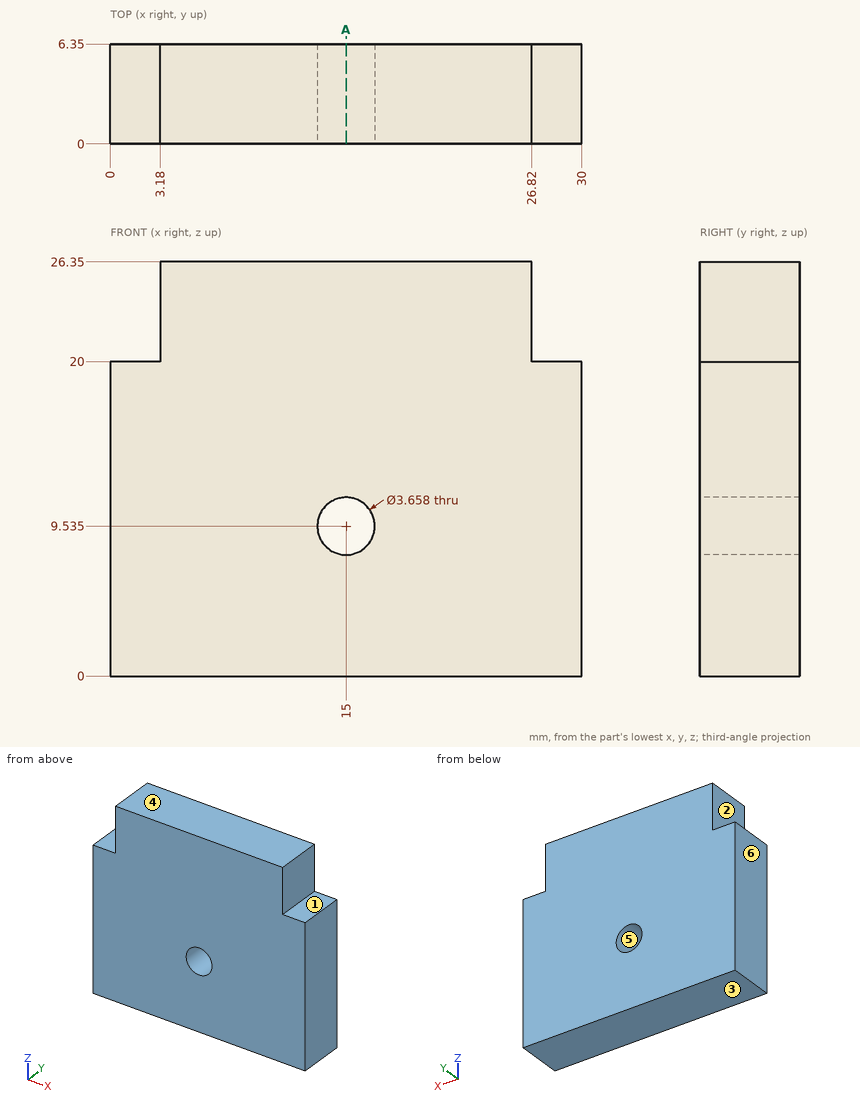
Drawing for the job (mm, zero at the part's lowest x, y, z). A direction names the side the tool comes from. Give positions to 0.01 mm unless a question says otherwise; leave off trailing zeros. Loops run counter-clockwise (first coordinate to the right, second up) from the corner with the lowest first, then second, coordinate; pieces in that order, holes last. Notation, with made-up numbers: (-28.5, 9.25) - (11.5, 9.25) arc R20 ccw to (11.5, 29.25) - close; hole circle Ø3 at (20.5, 33.5). An arc over 180 degrees is marked (long way). Write item = value, one per line. Start each with the question number.
1) Probe probe 1 along Z at (x, y) = (15, 1.5); probe 2 along X at (y, z) = (4.25, 24). List the from-to ranges inside material, lowest first. Write a range as from..to.
2) Pull direction Z, two halves, no side cores. Call the marked faces 4, 5 and 6: +Z half, -Z half, draft (parallel to the pull), parting line (faces both ways), or undercut.
3) Band-saw the part on A-A on x = 15. Give the cut face in (y, z).
4) Tool access for the marked faces 1, 2 and 3: list every direction of +Z, -Z, +X, -X, +Y, -Y with a clear straight run to the whole face (end or side of a thin tool).
5) Drop flat-ended pins along their axis: pin 1 Ø1 at (x, y) = (29, 3.5) entering from +Z; pin 2 Ø1.5 at (y, z) = (1.5, 21) entering from +X; pin 3 Ø1.9 at (y, z) = (3, 24.5) entering from -X. Give the stop position or say it passes through.
Final values:
q1.probe_1 = 0..7.71, 11.36..26.35
q1.probe_2 = 3.18..26.82
q2.face_4 = +Z half
q2.face_5 = undercut
q2.face_6 = draft
q3.outline = (0, 0) - (6.35, 0) - (6.35, 7.71) - (0, 7.71) - close; (0, 11.36) - (6.35, 11.36) - (6.35, 26.35) - (0, 26.35) - close
q4.face_1 = +Z, +X, +Y, -Y
q4.face_2 = +Z, -X, +Y, -Y
q4.face_3 = -Z, +X, -X, +Y, -Y
q5.pin_1 = 20
q5.pin_2 = 26.82
q5.pin_3 = 3.18
